For this review, take the finished solid that the model builds, in its own axes (mm). Face numbers are marked on the shaded views. A direction names the side the tool comes from. Give positions to 0.01 mm unless a question says otherwise; leave off trailing zeros. Loops run counter-clockwise (first coordinate to the right, second up) from the corner with the lowest first, then second, coordinate; pieces in that order, holes last. Notation, with made-up numbers: (75, 19.5) - (121, 19.5) arc R17 ccw to (121, 39.5) - close; hole circle Ø3 at (45.25, 65). An arc over 180 degrees is marked (long way). Use CSV: the item, a comma, the result in double quotes. Start each with the question number.
1. Take a section at A-A on y = 21.5. Give the boundary of the cut face in (x, z).
2. Take a section at B-B on z = 5. Give the boundary of the cut face in (x, y) (3 decimals), plus the area to 3 significant figures.
3. For pin 1 (4 mm diameter, centred on y = 6.5, z = 3.5, fed in from +X); pin 2 (5 mm diameter, centred on x = 24, z = 5.5, fed in from +Y); pin 3 (0.6 mm diameter, centred on y = 3.5, z = 1.5, fed in from +X), all flat-tipped, find the tip position at first contact; note any pin that passes through.
4. Wall thickness on line 1 (Y direction, x = 9.5, z = 0.4); line 2 (Z direction, x = 23.5, y = 20.5); line 3 (Z direction, x = 16, y = 8.75): over which ranges is each line inside the solid? List them lowest first.
5. Take a section at C-C on x = 35.5. Give the boundary of the cut face in (y, z).
6. For the marked faces 3, 4, 5 and 6, list the 3-axis set-ups (+Z, -Z, +X, -X, +Y, -Y) from which the entire face can be reached by the end or side of a thin tool; tool diameter is ignored.
7. Mouldability with a two-part tool opening along X and no side actions: class the marked faces 1 and 2 as pulls with the +X half, pulls with the -X half, needs draft (parallel to the pull), parting line crosses it, or undercut.
8. Take a section at D-D on y = 5.75. Give the boundary of the cut face in (x, z).
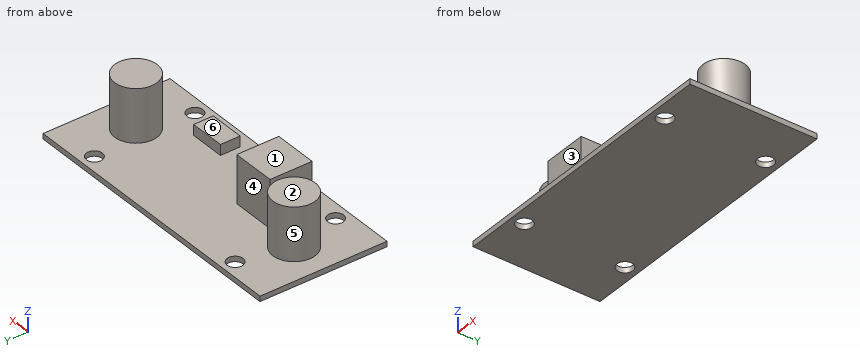
```python
from build123d import *

# Parameters (mm, degrees)
SKETCH1_W           = 54
SKETCH1_H           = 24
SKETCH1_R           = 1.5
SKETCH1_R_2         = 4
SKETCH1_W_2         = 6.671328762
SKETCH1_H_2         = 3.736160039
SKETCH1_W_3         = 8.286492568
SKETCH1_H_3         = 7.940799873
BOSS_EXTRUDE1_DEPTH = 1
SKETCH1_2_R         = 4
BOSS_EXTRUDE2_DEPTH = 11
SKETCH1_3_W         = 8.286492568
SKETCH1_3_H         = 7.940799873
BOSS_EXTRUDE3_DEPTH = 10
SKETCH1_4_W         = 6.671328762
SKETCH1_4_H         = 3.736160039
BOSS_EXTRUDE4_DEPTH = 3


with BuildPart() as part:
    # Sketch1 → Boss-Extrude1 (new body)
    with BuildSketch(Plane.XY):
        with Locations((27, 12)):
            Rectangle(SKETCH1_W, SKETCH1_H)
        with Locations((9.5, 21.5)):
            Circle(SKETCH1_R, mode=Mode.SUBTRACT)
        with Locations((9.5, 2.5)):
            Circle(SKETCH1_R, mode=Mode.SUBTRACT)
        with Locations(Location((44.5, 2.5, 0), (0, 0, 180))):
            Circle(SKETCH1_R, mode=Mode.SUBTRACT)
        with Locations(Location((44.5, 21.5, 0), (0, 0, 180))):
            Circle(SKETCH1_R, mode=Mode.SUBTRACT)
        with Locations((7.325006642, 12)):
            Circle(SKETCH1_R_2, mode=Mode.SUBTRACT)
        with Locations(Location((46.674993358, 12, 0), (0, 0, 180))):
            Circle(SKETCH1_R_2, mode=Mode.SUBTRACT)
        with Locations((36.573516425, 4.36808002)):
            Rectangle(SKETCH1_W_2, SKETCH1_H_2, mode=Mode.SUBTRACT)
        with Locations((17.437336555, 8.029600064)):
            Rectangle(SKETCH1_W_3, SKETCH1_H_3, mode=Mode.SUBTRACT)
    extrude(amount=BOSS_EXTRUDE1_DEPTH)

    # Sketch1_2 → Boss-Extrude2 (add)
    with BuildSketch(Plane.XY):
        with Locations((7.325006642, 12)):
            Circle(SKETCH1_2_R)
        with Locations(Location((46.674993358, 12, 0), (0, 0, 180))):
            Circle(SKETCH1_2_R)
    extrude(amount=BOSS_EXTRUDE2_DEPTH)

    # Sketch1_3 → Boss-Extrude3 (add)
    with BuildSketch(Plane.XY):
        with Locations((17.437336555, 8.029600064)):
            Rectangle(SKETCH1_3_W, SKETCH1_3_H)
    extrude(amount=BOSS_EXTRUDE3_DEPTH)

    # Sketch1_4 → Boss-Extrude4 (add)
    with BuildSketch(Plane.XY):
        with Locations((36.573516425, 4.36808002)):
            Rectangle(SKETCH1_4_W, SKETCH1_4_H)
    extrude(amount=BOSS_EXTRUDE4_DEPTH)


solid = part.part
```
Check result:
1,outline,"(0, 0) - (8, 0) - (8, 1) - (0, 1) - close; (11, 0) - (43, 0) - (43, 1) - (11, 1) - close; (46, 0) - (54, 0) - (54, 1) - (46, 1) - close"
2,outline,"circle Ø8 at (7.325, 12); (13.294, 4.059) - (21.581, 4.059) - (21.581, 12) - (13.294, 12) - close; circle Ø8 at (46.675, 12)"
2,area,"166 mm²"
3,pin 1,"stops at x = 48.61"
3,pin 2,"stops at y = 12"
3,pin 3,"stops at x = 39.91"
4,line 1,"y = 0 to 1, 4 to 20, 23 to 24"
4,line 2,"z = 0 to 1"
4,line 3,"z = 0 to 10"
5,outline,"(0, 0) - (24, 0) - (24, 1) - (6.24, 1) - (6.24, 3) - (2.5, 3) - (2.5, 1) - (0, 1) - close"
6,face 3,"+Z, -X, -Y"
6,face 4,"+Z, +Y"
6,face 5,"+Z"
6,face 6,"+Z, +X, +Y, -Y"
7,face 1,"undercut"
7,face 2,"needs draft"
8,outline,"(0, 0) - (54, 0) - (54, 1) - (39.91, 1) - (39.91, 3) - (33.24, 3) - (33.24, 1) - (21.58, 1) - (21.58, 10) - (13.29, 10) - (13.29, 1) - (0, 1) - close"
